Build history of the part. All positions in model axes, mm. Give positions to 0.01 mm unless a question says otherwise; leave off trailing zeros. Write item = value, one per line. Start each with the question number.
from build123d import *

# Parameters (mm, degrees)
SKETCH2_W                                  = 95
SKETCH2_H                                  = 107
SKETCH2_R                                  = 2
BOSS_EXTRUDE1_DEPTH                        = 3
SKETCH7_R                                  = 1
CUT_EXTRUDE2_DEPTH                         = 10
MIRROR3_COPY_1_SKETCH_R                    = 1
MIRROR3_COPY_1_DEPTH                       = 10
MIRROR3_AT_THE_SECOND_PLANE_COPY_1_SKETC_R = 1
MIRROR3_AT_THE_SECOND_PLANE_COPY_1_DEPTH   = 10
MIRROR3_AT_THE_SECOND_PLANE_COPY_2_SKETC_R = 1
MIRROR3_AT_THE_SECOND_PLANE_COPY_2_DEPTH   = 10
MIRROR3_AT_THE_SECOND_PLANE_COPY_3_SKETC_R = 1
MIRROR3_AT_THE_SECOND_PLANE_COPY_3_DEPTH   = 10


with BuildPart() as part:
    # Sketch2 → Boss-Extrude1 (new body)
    with BuildSketch(Plane(origin=(0, 0, 0), x_dir=(1, 0, 0), z_dir=(0, 1, 0))):
        Rectangle(SKETCH2_W, SKETCH2_H)
        with Locations(Location((38.075, -43.825, 0), (0, 0, 270))):
            Circle(SKETCH2_R, mode=Mode.SUBTRACT)
        with Locations(Location((38.075, 43.825, 0), (0, 0, 270))):
            Circle(SKETCH2_R, mode=Mode.SUBTRACT)
        with Locations(Location((-38.075, -43.825, 0), (0, 0, 270))):
            Circle(SKETCH2_R, mode=Mode.SUBTRACT)
        with Locations(Location((-38.075, 43.825, 0), (0, 0, 270))):
            Circle(SKETCH2_R, mode=Mode.SUBTRACT)
    extrude(amount=BOSS_EXTRUDE1_DEPTH)

    # Sketch7 → Cut-Extrude2 (cut)
    with BuildSketch(Plane(origin=(0, 3, 0), x_dir=(1, 0, 0), z_dir=(0, 1, 0))):
        with Locations(Location((42.63, 46.04, 0), (0, 0, 270))):
            Circle(SKETCH7_R)
    cut_extrude2 = extrude(amount=-CUT_EXTRUDE2_DEPTH, mode=Mode.SUBTRACT)

    # Mirror2: Cut-Extrude2 across plane
    add(cut_extrude2.mirror(Plane(origin=(0, 0, -28.738611276), x_dir=(1, 0, 0), z_dir=(0, 0, -1))), mode=Mode.SUBTRACT)

    # Mirror3: Cut-Extrude2 across plane
    add(cut_extrude2.mirror(Plane(origin=(0, 0, 0), x_dir=(0, 0, 1), z_dir=(1, 0, 0))), mode=Mode.SUBTRACT)

    # Mirror3 copy 1 sketch → Mirror3 copy 1 (cut)
    with BuildSketch(Plane(origin=(0, 3, -57.477222552), x_dir=(-1, 0, 0), z_dir=(0, 1, 0))):
        with Locations(Location((42.63, 46.04, 0), (0, 0, 270))):
            Circle(MIRROR3_COPY_1_SKETCH_R)
    extrude(amount=-MIRROR3_COPY_1_DEPTH, mode=Mode.SUBTRACT)

    # Mirror3 at the second plane: Cut-Extrude2 across plane
    add(cut_extrude2.mirror(Plane.XY), mode=Mode.SUBTRACT)

    # Mirror3 at the second plane copy 1 sketc → Mirror3 at the second plane copy 1 (cut)
    with BuildSketch(Plane(origin=(0, 3, 57.477222552), x_dir=(1, 0, 0), z_dir=(0, 1, 0))):
        with Locations(Location((42.63, 46.04, 0), (0, 0, 270))):
            Circle(MIRROR3_AT_THE_SECOND_PLANE_COPY_1_SKETC_R)
    extrude(amount=-MIRROR3_AT_THE_SECOND_PLANE_COPY_1_DEPTH, mode=Mode.SUBTRACT)

    # Mirror3 at the second plane copy 2 sketc → Mirror3 at the second plane copy 2 (cut)
    with BuildSketch(Plane(origin=(0, 3, 0), x_dir=(-1, 0, 0), z_dir=(0, 1, 0))):
        with Locations(Location((42.63, 46.04, 0), (0, 0, 270))):
            Circle(MIRROR3_AT_THE_SECOND_PLANE_COPY_2_SKETC_R)
    extrude(amount=-MIRROR3_AT_THE_SECOND_PLANE_COPY_2_DEPTH, mode=Mode.SUBTRACT)

    # Mirror3 at the second plane copy 3 sketc → Mirror3 at the second plane copy 3 (cut)
    with BuildSketch(Plane(origin=(0, 3, 57.477222552), x_dir=(-1, 0, 0), z_dir=(0, 1, 0))):
        with Locations((42.63, -46.04)):
            Circle(MIRROR3_AT_THE_SECOND_PLANE_COPY_3_SKETC_R)
    extrude(amount=-MIRROR3_AT_THE_SECOND_PLANE_COPY_3_DEPTH, mode=Mode.SUBTRACT)


solid = part.part
(1) Mould opens along Z. For faces 1 (the face through (-1, 1, 53.5)), 2 (the face through (37.309, 1.479, -41.978)), 3 (the face through (-1, 3, -1)) say: released by +Z, released by -Z, zero draft, split by the parting line, or undercut.
(2) Flat gauge pin, fed straight in: P1, Ø1.8, axis at x = -42.63, z = -46.04, coming from the +Y side. Where does the tip first touch, or does it go through?
(3) Wall check: line 1 (X direction, y = 0.85, z = -46.04); line 2 (Z direction, x = -38, y = 2.35); line 3 (Z direction, x = -42.63, y = 2.35). Give the ranges that are in metal, low to high. Write a range as [from, to].
Results:
q1.face_1 = released by +Z
q1.face_2 = undercut
q1.face_3 = zero draft
q2.P1 = through
q3.line_1 = [-47.5, -43.63], [-41.63, 41.63], [43.63, 47.5]
q3.line_2 = [-53.5, -45.82], [-41.83, 41.83], [45.82, 53.5]
q3.line_3 = [-53.5, -47.04], [-45.04, -12.44], [-10.44, 10.44], [12.44, 45.04], [47.04, 53.5]
